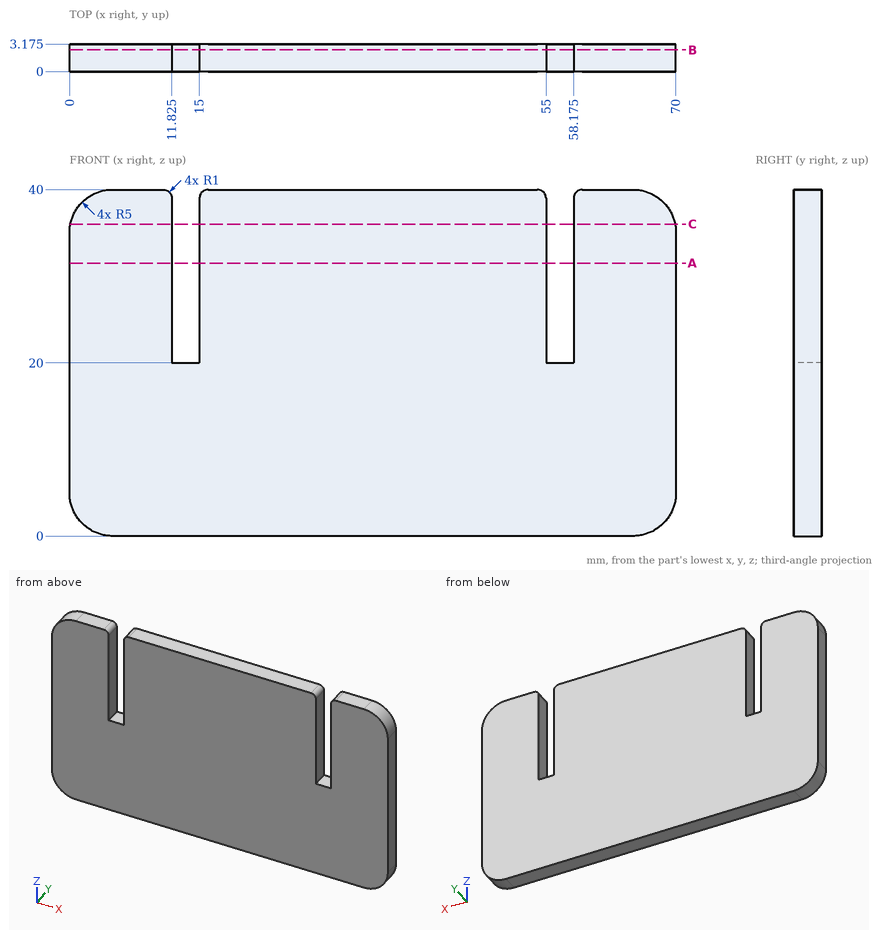
Geometry: see drawing. Coordinates: mm, zero at the bounding-box minimum. Round coordinates to 2 decimals unless told otherwise and drop trailing zeros. Loops run counter-clockwise (first coordinate to the right, second up) from the corner with the lowest first, then second, coordinate; pieces in that order, holes last. Notation, with made-up numbers: M 4,-30.5 L 50,-30.5 A20 ccw 50,8.5 Z; hole C 54,-37 d11. An arc over 180 degrees is marked long. Use a Markdown table: item, result. Add a question column.
1. Section query A-A on z = 31.5. Return the cut outline in (x, y) (3 decimals), then the cut area to 3 significant figures.
2. Section query C-C on z = 36. Return the cut outline in (x, y) (3 decimals), then the cut area to 3 significant figures.
3. Section query B-B on y = 2.5. Return the cut outline in (x, z) (3 decimals).
4. Line query: line 1 (X direction, y = 1.85, z = 21.5) (3 decimals); line 2 (X direction, y = 1.4, z = 36) (3 decimals); line 3 (Z direction, x = 13, y = 1.15). Output: solid intervals per line, ascending.
Reported:
| question | item | result |
|---|---|---|
| 1 | outline | M 0,0 L 11.825,0 L 11.825,3.175 L 0,3.175 Z; M 15,0 L 55,0 L 55,3.175 L 15,3.175 Z; M 58.175,0 L 70,0 L 70,3.175 L 58.175,3.175 Z |
| 1 | area | 202 mm² |
| 2 | outline | M 0.101,0 L 11.825,0 L 11.825,3.175 L 0.101,3.175 Z; M 15,0 L 55,0 L 55,3.175 L 15,3.175 Z; M 58.175,0 L 69.899,0 L 69.899,3.175 L 58.175,3.175 Z |
| 2 | area | 201 mm² |
| 3 | outline | M 0,5 A5 ccw 5,0 L 65,0 A5 ccw 70,5 L 70,35 A5 ccw 65,40 L 59.175,40 A1 ccw 58.175,39 L 58.175,20 L 55,20 L 55,39 A1 ccw 54,40 L 16,40 A1 ccw 15,39 L 15,20 L 11.825,20 L 11.825,39 A1 ccw 10.825,40 L 5,40 A5 ccw 0,35 Z |
| 4 | line 1 | x = 0 to 11.825, 15 to 55, 58.175 to 70 |
| 4 | line 2 | x = 0.101 to 11.825, 15 to 55, 58.175 to 69.899 |
| 4 | line 3 | z = 0 to 20 |
